Source: CAD feature listing. Evaluate the final solid. Frame: model axes, mm. A direction names the side the tool comes from. Give positions to 0.01 mm unless a question says otherwise; leave off trailing zeros. Write each loop counter-clockwise with the first axis right and the second up, starting at its lowest first coordinate (ties: lowest second). Pieces come first, ordered by that corner, then holes.
Autodesk Inventor part; units mm, degrees
ref_plane "YZ Plane" through (0, 0, 0) normal (1, 0, 0) x (0, 1, 0)
ref_plane "XZ Plane" through (0, 0, 0) normal (0, 1, 0) x (-1, 0, 0)
ref_plane "XY Plane" through (0, 0, 0) normal (0, 0, 1) x (1, 0, 0)
sketch "Sketch1" plane through (0, 0, 0) normal (0, 0, 1) x (1, 0, 0)
  line L0 (6, 5) -> (6, 13)
  line L1 (0, 16) -> (0, 0)
  arc A0 (37.0043, 34) -> (18.539, 41.6832) centre (26.1732, 34) ccw
  line L2 (18.539, 41.6832) -> (0, 16)
  circle A1 centre (26.1732, 34) radius 2
  line L3 (37.0043, 5) -> (37.0043, 0)
  line L4 (6, 5) -> (37.0043, 5)
  line L5 (0, 0) -> (37.0043, 0)
  line L6 (6, 13) -> (37.0043, 13)
  line L7 (0, 16) -> (37.0043, 16)
  line L8 (37.0043, 34) -> (37.0043, 13)
  dimension "d3" = 8
  dimension "d6" = 18
  dimension "d7" = 20
  dimension "d8" = 4
  dimension "d9" = 3
  dimension "d10" = 5
  dimension "d11" = 16
  dimension "d12" = 37.0043
  dimension "d13" = 31.0043
  dimension "d14" = 26.1732
extrude "Extrusion1" add sketch "Sketch1" along normal blind 26
sketch "Sketch2" plane through (0, 0, 26) normal (0, 0, 1) x (1, 0, 0)
  point P0 (0, 0)
sketch "Sketch3" plane through (37.0043, 13, 0) normal (1, 0, 0) x (0, 0, -1)
  line L0 (0, 0) -> (-26, 0)
  line L1 (-13, 38) -> (-3.75, 38)
  line L2 (-3.75, 38) -> (-3.75, 3)
  line L3 (-13, 38) -> (-22.25, 38)
  line L4 (-22.25, 38) -> (-22.25, 3)
  line L5 (-22.25, 3) -> (-3.75, 3)
  line L6 (0, 0) -> (-26, 0)
  point P0 (0, -13)
  point P1 (-26, 3)
  dimension "d19" = 9.25
  dimension "d20" = 9.25
extrude "Extrusion2" cut sketch "Sketch3" against normal through all
properties part number "Maintients poullies V2 alpha"
1. Mould query, pull axis X, two halves, no side actions, for faces 4 (the flat face through (9.4, 29.02, 1.85)), 5 (the flat face through (21, 5, 13)), 6 (the cylindrical face through (25.74, 35.952, 24.099)). Classes: +X half, -X half, draft (parallel to the pull), parting line (faces both ways), or undercut.
2. Cut plane C-C, the plane z = 1.5. Return the cut outline in (x, y).
3. Cut plane B-B, the plane x = 31.5. Return the cut outline in (y, z), then the cut area to 3 significant figures.
4. Cut plane A-A, the plane y = 23. Return the cut outline in (x, z).
5. Cut plane D-D, the plane z = 16.75. Return the cut outline in (x, y), then the cut area to 3 significant figures.
6. Contact query for flat-ended pins moving along their axis: P1, Ø8, axis at x = 14, z = 14, coming from the +Y side; P2, Ø3, axis at y = 9, z = 17, coming from the +X side. Output: stop coordinate, or through.
7. Line query: L1, parallel to Z at x = 32, y = 39; L2, parallel to X at y = 34, z = 1.6; L3, parallel to Y at x = 33.5, z = 14.5. Output: solid intervals per line, ascending.
8. Access query for faces 1 (the flat face through (18, 23, 0)), 2 (the flat face through (23, 27, 22.25)), 3 (the flat face through (21, 13, 13)). Directions: +Z, -Z, +X, -X, +Y, -Y. A direction counts if a zero-diameter tool reaches every point of the face in a straight line with its end or side. Return the directions, or none.
Response values:
1. face 4: -X half
1. face 5: draft
1. face 6: undercut
2. outline: (0, 0) - (37, 0) - (37, 5) - (6, 5) - (6, 13) - (37, 13) - (37, 34) arc R10.83 ccw to (18.54, 41.68) - (0, 16) - close; hole circle Ø4 at (26.17, 34)
3. outline: (0, 0) - (5, 0) - (5, 26) - (0, 26) - close; (13, 0) - (43.43, 0) - (43.43, 3.75) - (16, 3.75) - (16, 22.25) - (43.43, 22.25) - (43.43, 26) - (13, 26) - close
3. area: 414 mm2
4. outline: (5.05, 0) - (37, 0) - (37, 3.75) - (5.05, 3.75) - close; (5.05, 22.25) - (37, 22.25) - (37, 26) - (5.05, 26) - close
5. outline: (0, 0) - (37, 0) - (37, 5) - (6, 5) - (6, 13) - (37, 13) - (37, 16) - (0, 16) - close
5. area: 344 mm2
6. P1: stops at y = 16
6. P2: stops at x = 6
7. L1: z = 0 to 3.75, 22.25 to 26
7. L2: x = 12.99 to 24.17, 28.17 to 37
7. L3: y = 0 to 5, 13 to 16
8. face 1: -Z, +X, -X, +Y, -Y
8. face 2: +X, -X, +Y
8. face 3: +Z, -Z, +X
